Design review of the part built by this model. Coordinates are the model's own, in mm. A direction names the side the tool comes from. Coordinates: 2 decimals unless noted, no trailing zeros. Order: outer loops, then holes, each group sorted by start corner. A loop starts at its lowest first (then second) coordinate and runs counter-clockwise, first axis right, second up.
from build123d import *

# Parameters (mm, degrees)
SKETCH1_R                = 8
BOSS_EXTRUDE1_DEPTH      = 32
SHELL3_START             = 2
SHELL3_OUTLINE_R         = 10
SHELL3_DEPTH             = 28
BOSS_EXTRUDE2_DEPTH      = 8
BOSS_EXTRUDE2_DEPTH_BACK = 40
SKETCH2_R                = 5
CHAMFER1_SIZE            = 2


# Read off the part's stored shape, not the designer's step: Shell3
with BuildPart() as part:
    # Sketch1 → Boss-Extrude1 (new body)
    with BuildSketch(Plane(origin=(0, 0, 0), x_dir=(1, 0, 0), z_dir=(0, 1, 0))):
        with BuildLine():
            Line((6, 84), (14, 62.745966692))
            Line((14, 62.745966692), (14, 7.745966692))
            ThreePointArc((14, 7.745966692), (-8.126024025, -13.782878275), (0, 16))
            Line((0, 16), (0, 84))
            Line((0, 84), (6, 84))
        make_face()
        with Locations(Location((0, 0, 0), (0, 0, 270))):
            Circle(SKETCH1_R, mode=Mode.SUBTRACT)
    extrude(amount=BOSS_EXTRUDE1_DEPTH)

    # Shell3 outline → Shell3 (cut)
    with BuildSketch(Plane(origin=(0, 0, 0), x_dir=(1, 0, 0), z_dir=(0, 1, 0)).offset(SHELL3_START)):
        with BuildLine():
            ThreePointArc((2, 15.874507866), (1.001966601, 15.968596148), (0, 16))
            ThreePointArc((0, 16), (-8.126024026, -13.782878275), (14, 7.745966692))
            ThreePointArc((14, 7.745966692), (13.077163184, 9.218882962), (12, 10.583005244))
            Line((12, 10.583005244), (12, 62.382030987))
            Line((12, 62.382030987), (4.615813204, 82))
            Line((4.615813204, 82), (2, 82))
            Line((2, 82), (2, 15.874507866))
        make_face()
        Circle(SHELL3_OUTLINE_R, mode=Mode.SUBTRACT)
    extrude(amount=SHELL3_DEPTH, mode=Mode.SUBTRACT)

    # Sketch2 → Boss-Extrude2 (add, two sides: drawn at the far end of the back side and taken through both)
    with BuildSketch(Plane(origin=(0, 32, 0), x_dir=(1, 0, 0), z_dir=(0, 1, 0)).offset(-BOSS_EXTRUDE2_DEPTH_BACK)):
        with Locations(Location((0, 84, 0), (0, 0, 270))):
            Circle(SKETCH2_R)
    extrude(amount=BOSS_EXTRUDE2_DEPTH + BOSS_EXTRUDE2_DEPTH_BACK)

    # Chamfer1
    chamfer1_edges = [part.edges().sort_by_distance(p)[0] for p in [
        (0, -8, -89),
        (0, 40, -89),
    ]]
    chamfer(chamfer1_edges, length=CHAMFER1_SIZE)


solid = part.part
1. Add section D-D (x = -12.5). Give the boundary of the cut face in (y, z), and give its area (3 significant figures).
2. Insertion check: pin 1 (5 mm diameter, centred on x = 10, z = -74, fed in from -Y); pin 2 (14 mm diameter, centred on y = 18, z = -55, fed in from +X); pin 3 (8 mm diameter, centred on y = 32.5, z = -69.5, fed in from -X). Each pin has a flat end and moves straight along its axis. Give the tip position at first contact, or say it passes through.
3. Mouldability with a two-part tool opening along Y and no side actions: class faces 5 (the flat face through (0, 40, -84)), 6 (the cylindrical face through (-7.81, 15.78, -1.73)), 7 (the flat face through (0, -8, -84)), 8 (the flat face through (2, 16, -48)) as pulls with the +Y half, pulls with the -Y half, needs draft (parallel to the pull), parting line crosses it, or undercut.
4. Add section A-A (y = 27.5). State how many separate pieces and enclosed holes the cut face has, and give its area (3 significant figures).
5. Add section C-C (z = -46.5). Give the boundary of the cut face in (x, y).
6. To check wall thickness, follow line 1 (X direction, y = 8, z = -16.5); line 2 (X direction, y = 24, z = 0); line 3 (Y direction, x = 7, z = -28). State the ranges of each line that lie inside material, in increasing order.
7. Add section B-B (z = 0). Give the boundary of the cut face in (x, y), and give its area (3 significant figures).
8. For faces 1 (the cylindrical face through (-2.17, 15.8, 9.76)), 2 (the flat face through (0, 16, -47)), 3 (the cylindrical face through (1.016, 15.804, -15.968)), 4 (the flat face through (12, 16, -36)), list the 3-axis set-ups (+Z, -Z, +X, -X, +Y, -Y) from which the entire face can be reached by the end or side of a thin tool; tool diameter is ignored.
Solution:
1. outline: (0, -9.99) - (2, -9.99) - (2, 9.99) - (0, 9.99) - close; (30, -9.99) - (32, -9.99) - (32, 9.99) - (30, 9.99) - close
1. area: 79.9 mm2
2. pin 1: stops at y = 0
2. pin 2: stops at x = 14
2. pin 3: stops at x = 0
3. face 5: pulls with the +Y half
3. face 6: needs draft
3. face 7: pulls with the -Y half
3. face 8: undercut
4. separate pieces: 2
4. enclosed holes: 1
4. area: 469 mm2
5. outline: (0, 0) - (14, 0) - (14, 32) - (0, 32) - close; hole (2, 2) - (12, 2) - (12, 30) - (2, 30) - close
6. line 1: x = 0 to 2, 12 to 14
6. line 2: x = -10 to -8, 8 to 10
6. line 3: y = 0 to 2, 30 to 32
7. outline: (-16, 0) - (-8, 0) - (-8, 32) - (-16, 32) - (-16, 30) - (-10, 30) - (-10, 2) - (-16, 2) - close; (8, 0) - (16, 0) - (16, 2) - (10, 2) - (10, 30) - (16, 30) - (16, 32) - (8, 32) - close
7. area: 176 mm2
8. face 1: none
8. face 2: -X, +Y, -Y
8. face 3: -X
8. face 4: +Z
